Input: part model. Units: mm. Frame: model coordinates. Face numbers are marked on the shaded views. A direction names the side the tool comes from. Coordinates: 2 decimals unless noted, no trailing zeros. Loops run counter-clockwise (first coordinate to the right, second up) from the corner with the lowest first, then second, coordinate; pieces in that order, holes last. Notation, with made-up numbers: (75, 25) - (133, 25) arc R9 ccw to (133, 34) - close; hole circle Ø10 at (65.5, 49). An arc over 180 degrees is marked (long way). Use one line per item in the form item = value.
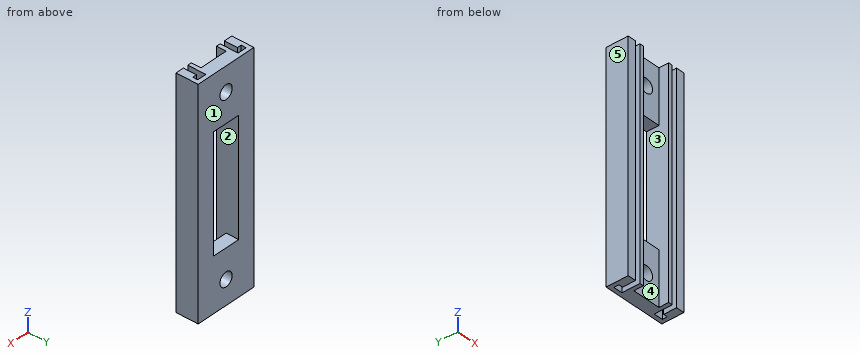
from build123d import *

# Parameters (mm, degrees)
BOSS_EXTRUDE1_DEPTH   = 160
BOSS_EXTRUDE1_2_DEPTH = 160
BOSS_EXTRUDE2_START   = 16
SKETCH3_W             = 20.6
SKETCH3_H             = 160
BOSS_EXTRUDE2_DEPTH   = 9
CUT_EXTRUDE1_START    = 16
SKETCH4_R             = 5
CUT_EXTRUDE1_DEPTH    = 9
CUT_EXTRUDE2_START    = 16
SKETCH5_W             = 20.6
SKETCH5_H             = 83
CUT_EXTRUDE2_DEPTH    = 9


with BuildPart() as part:
    # Sketch2 → Boss-Extrude1 (new body)
    with BuildSketch(Plane.XY):
        Polygon((0, 0), (0, 9.4), (-3, 9.4), (-3, 13), (3.6, 13), (3.6, 0), (6.5, 0), (6.5, 16), (-6, 16), (-6, 0), align=None)
    extrude(amount=BOSS_EXTRUDE1_DEPTH)



with BuildPart() as body_2:
    # Sketch2 → Boss-Extrude1 2 (new body)
    with BuildSketch(Plane.XY):
        Polygon((39.6, 0), (33.6, 0), (33.6, 9.4), (36.6, 9.4), (36.6, 13), (30, 13), (30, 0), (27.1, 0), (27.1, 16), (39.6, 16), align=None)
    extrude(amount=BOSS_EXTRUDE1_2_DEPTH)


with BuildPart() as part_1:
    add(part.part)

    add(body_2.part)  # Boss-Extrude2 merges body 2
    # Sketch3 → Boss-Extrude2 (add)
    with BuildSketch(Plane(origin=(0, 0, 0), x_dir=(1, 0, 0), z_dir=(0, 1, 0)).offset(BOSS_EXTRUDE2_START)):
        with Locations((16.8, -80)):
            Rectangle(SKETCH3_W, SKETCH3_H)
    extrude(amount=-BOSS_EXTRUDE2_DEPTH)

    # Sketch4 → Cut-Extrude1 (cut)
    with BuildSketch(Plane(origin=(0, 0, 0), x_dir=(1, 0, 0), z_dir=(0, 1, 0)).offset(CUT_EXTRUDE1_START)):
        with Locations((16.8, -17.5)):
            Circle(SKETCH4_R)
        with Locations((16.8, -142.5)):
            Circle(SKETCH4_R)
    extrude(amount=-CUT_EXTRUDE1_DEPTH, mode=Mode.SUBTRACT)

    # Sketch5 → Cut-Extrude2 (cut)
    with BuildSketch(Plane(origin=(0, 0, 0), x_dir=(1, 0, 0), z_dir=(0, 1, 0)).offset(CUT_EXTRUDE2_START)):
        with Locations((16.8, -80)):
            Rectangle(SKETCH5_W, SKETCH5_H)
    extrude(amount=-CUT_EXTRUDE2_DEPTH, mode=Mode.SUBTRACT)


solid = part_1.part
Q1. Cut plane A-A, the plane x = 16.8. Return loops of the section in (y, z), then the cut area to 3 significant figures.
Check values:
outline = (7, 0) - (16, 0) - (16, 12.5) - (7, 12.5) - close; (7, 22.5) - (16, 22.5) - (16, 38.5) - (7, 38.5) - close; (7, 121.5) - (16, 121.5) - (16, 137.5) - (7, 137.5) - close; (7, 147.5) - (16, 147.5) - (16, 160) - (7, 160) - close
area = 513 mm²
Q2. Pull-direction query (Z, two-part tool) for the marked faces 1, 2 and 3; classes: pulls with the +Z half, pulls with the -Z half, needs draft (parallel to the pull), parting line crosses it, or undercut.
Check values:
face_1 = needs draft
face_2 = undercut
face_3 = undercut
Q3. Set-up query: the marked faces 4 and 5. Return all of +Z, -Z, +X, -X, +Y, -Y with unobstructed straight access to the full face (end or side cutting, diameter ignored); none if empty.
Check values:
face_4 = +Z, -Z, -Y
face_5 = +Z, -Z, -X, +Y, -Y
Q4. Ray query, line 1 along X through (y, z) = (12.25, 17.5); line 2 along Z through (x, y) = (16.8, 14); line 3 along X through (y, z) = (5, 16.5). Return the intervals inside material, ascending. Write a range as [from, to].
Check values:
line_1 = [-6, -3], [3.6, 11.8], [21.8, 30], [36.6, 39.6]
line_2 = [0, 12.5], [22.5, 38.5], [121.5, 137.5], [147.5, 160]
line_3 = [-6, 0], [3.6, 6.5], [27.1, 30], [33.6, 39.6]
Q5. Cut plane B-B, the plane z = 73.5. Return loops of the section in (x, y), then the cut area to 3 significant figures.
Check values:
outline = (-6, 0) - (0, 0) - (0, 9.4) - (-3, 9.4) - (-3, 13) - (3.6, 13) - (3.6, 0) - (6.5, 0) - (6.5, 16) - (-6, 16) - close; (27.1, 0) - (30, 0) - (30, 13) - (36.6, 13) - (36.6, 9.4) - (33.6, 9.4) - (33.6, 0) - (39.6, 0) - (39.6, 16) - (27.1, 16) - close
area = 285 mm²
Q6. Cut plane C-C, the plane z = 142.5. Return loops of the section in (x, y), then the cut area to 3 significant figures.
Check values:
outline = (-6, 0) - (0, 0) - (0, 9.4) - (-3, 9.4) - (-3, 13) - (3.6, 13) - (3.6, 0) - (6.5, 0) - (6.5, 7) - (11.8, 7) - (11.8, 16) - (-6, 16) - close; (21.8, 7) - (27.1, 7) - (27.1, 0) - (30, 0) - (30, 13) - (36.6, 13) - (36.6, 9.4) - (33.6, 9.4) - (33.6, 0) - (39.6, 0) - (39.6, 16) - (21.8, 16) - close
area = 380 mm²
Q7. First-contact query: P1, Ø16.5, axis at x = 17, z = 11.5, coming from the -Y side; P2, Ø1, axis at x = 32.5, z = 43, coming from the -Y side. Flat tips, straight axial feed; report the tip coordinate or a pass-through.
Check values:
P1 = 7
P2 = 13
